Read the model definition and answer for the solid it produces. Units are mm, in the model's axes. A direction names the side the tool comes from. Coordinates: 2 decimals unless noted, no trailing zeros. Order: outer loops, then holes, each group sorted by start corner. A loop starts at its lowest first (then second) coordinate and runs counter-clockwise, first axis right, second up. Notation, with made-up numbers: (17.25, 23.25) -> (33.25, 23.25) arc R13 ccw to (33.25, 47.25) -> close; hole circle Ø5 at (34, 83.5). An arc over 180 degrees is marked (long way). Use CSV: the item, a comma, the result in double quotes.
Autodesk Inventor part; units mm, degrees
ref_plane "YZ Plane" through (0, 0, 0) normal (1, 0, 0) x (0, 1, 0)
ref_plane "XZ Plane" through (0, 0, 0) normal (0, 1, 0) x (-1, 0, 0)
ref_plane "XY Plane" through (0, 0, 0) normal (0, 0, 1) x (1, 0, 0)
sketch "スケッチ1" plane through (0, 0, 0) normal (0, 1, 0) x (-1, 0, 0)
  line L0 (15.25, 10) -> (-15.25, 10)
  line L1 (-15.25, 10) -> (-15.25, -10)
  line L2 (-15.25, -10) -> (15.25, -10)
  line L3 (15.25, -10) -> (15.25, 10)
  line L4 (15.25, 10) -> (-15.25, -10) construction
  line L5 (-15.25, 10) -> (15.25, -10) construction
  line L6 (12.25, -8) -> (-12.25, -8)
  line L7 (-12.25, -8) -> (-12.25, 8)
  line L8 (-12.25, 8) -> (12.25, 8)
  line L9 (12.25, 8) -> (12.25, -8)
  circle A0 centre (-16.25, -5) radius 1.1
  line L10 (-15.25, 0) -> (15.25, 0) construction
  line L11 (0, 0) -> (0, -10) construction
  circle A1 centre (-16.25, 5) radius 1.1
  circle A2 centre (16.25, -5) radius 1.1
  circle A3 centre (16.25, 5) radius 1.1
  point P0 (0, 0)
  point P1 (-15.25, 5.4583)
  point P2 (-15.25, 4.5417)
  point P3 (-15.25, -4.5417)
  point P4 (-15.25, -5.4583)
  point P5 (15.25, -5.4583)
  point P6 (15.25, -4.5417)
  point P7 (15.25, 4.5417)
  point P8 (15.25, 5.4583)
  dimension "d0" = 30.5
  dimension "d1" = 20
  dimension "d3" = 2.2
  dimension "d4" = 1
  dimension "d5" = 10
  dimension "d16" = 2
  dimension "d17" = 2
  dimension "d18" = 3
  dimension "d19" = 3
extrude "押し出し1" add sketch "スケッチ1" along normal blind 3 contours L3 A3 A2 L2 L1 A0 A1 L0
fillet "フィレット1" radius 2 4 edges at (12.25, 1.5, -8) (12.25, 1.5, 8) (-12.25, 1.5, 8) (-12.25, 1.5, -8)
sketch "スケッチ2" plane through (-15.25, 0, -4.5417) normal (-1, 0, 0) x (0, 0, 1)
  line L0 (10.5417, 3) -> (10.5417, 0)
  line L1 (-1.4583, 0) -> (-1.4583, 3)
  line L2 (-1.4583, 3) -> (-1.4583, 0)
  line L3 (-0.9165, 0) -> (0, 0)
  line L4 (-1.4583, 3) -> (-1.4583, 0)
  line L5 (-0.9165, 0) -> (0, 0)
  line L6 (9.0835, 0) -> (10, 0)
  line L7 (10.5417, 0) -> (10.5417, 3)
  point P0 (4.5417, 0)
  point P1 (9.5417, 1.5)
  point P2 (-0.4583, 1.5)
  point P3 (-1.4583, 1.5)
  point P4 (-0.4583, 0)
  point P5 (9.5417, 0)
  point P6 (10.5417, 1.5)
hole "穴1" at (-15.25, 1.5, 5) at (-15.25, 1.5, -5) direction (1, 0, 0) diameter 1.567 end through all
equation "\"d17\" = d16"
equation "\"d19\" = d18"
properties part number "free_suzikai" material "アルミニウム 2014-T4"
Item 1: Find section D-D, the plane z = 5. Give the vertices of the cut face in (x, y), then the cut area to 3 significant figures.
Return value:
outline,"(-15.15, 0) -> (-12.25, 0) -> (-12.25, 0.72) -> (-15.15, 0.72) -> close; (-15.15, 2.28) -> (-12.25, 2.28) -> (-12.25, 3) -> (-15.15, 3) -> close; (12.25, 0) -> (15.15, 0) -> (15.15, 0.72) -> (12.25, 0.72) -> close; (12.25, 2.28) -> (15.15, 2.28) -> (15.15, 3) -> (12.25, 3) -> close"
area,"8.31 mm^2"
Item 2: Find section B-B, the plane x = 4. Give the vertices of the cut face in (y, z).
Return value:
outline,"(0, -10) -> (3, -10) -> (3, -8) -> (0, -8) -> close; (0, 8) -> (3, 8) -> (3, 10) -> (0, 10) -> close"
Item 3: The mould has two halves that part along Z. Classify faces 1 (the cylindrical face through (13.771, 1.8, 5.724)), 2 (the flat face through (15.25, 1, 8)), 3 (the flat face through (0, 1, 10)): +Z half, -Z half, draft (parallel to the pull), parting line (faces both ways), or undercut.
Return value:
face 1,"undercut"
face 2,"draft"
face 3,"+Z half"
Item 4: Find section A-A, the plane z = 0.75. Give the vertices of the cut face in (x, y).
Return value:
outline,"(-15.25, 0) -> (-12.25, 0) -> (-12.25, 3) -> (-15.25, 3) -> close; (12.25, 0) -> (15.25, 0) -> (15.25, 3) -> (12.25, 3) -> close"
Item 5: Find section C-C, the plane y = 2.7. Give the vertices of the cut face in (x, z), then the cut area to 3 significant figures.
Return value:
outline,"(-15.25, -10) -> (15.25, -10) -> (15.25, -5.46) arc R1.1 cw to (15.25, -4.54) -> (15.25, 4.54) arc R1.1 cw to (15.25, 5.46) -> (15.25, 10) -> (-15.25, 10) -> (-15.25, 5.46) arc R1.1 cw to (-15.25, 4.54) -> (-15.25, -4.54) arc R1.1 cw to (-15.25, -5.46) -> close; hole (-12.25, -6) arc R2 ccw to (-10.25, -8) -> (10.25, -8) arc R2 ccw to (12.25, -6) -> (12.25, 6) arc R2 ccw to (10.25, 8) -> (-10.25, 8) arc R2 ccw to (-12.25, 6) -> close"
area,"221 mm^2"
Item 6: A tool of negligible diameter and unlimited length cuts with its end or side. For faces 4 (the flat face through (0, 1, -10)), 5 (the flat face through (0, 1, -8)), from which of +Z, -Z, +X, -X, +Y, -Y can it reach the whole face along a straight path? Write none if from no direction.
Return value:
face 4,"-Z, +X, -X, +Y, -Y"
face 5,"+Y, -Y"
Item 7: Straight lines are drawn through the part: line 1 along Z through (x, y) = (14.45, 1.5); line 2 along X through (y, z) = (1.65, 2.75); line 3 along Y through (x, z) = (-13.6, -5). For each, find the intervals that lie inside material, in ascending order.
Return value:
line 1,"z = -10 to -5.78, -4.22 to 4.22, 5.78 to 10"
line 2,"x = -15.25 to -12.25, 12.25 to 15.25"
line 3,"y = 0 to 0.72, 2.28 to 3"
